Build history of the part. All positions in model axes, mm. A direction names the side the tool comes from. Coordinates: 2 decimals unless noted, no trailing zeros. Write each loop counter-clockwise with the first axis right and the second up, starting at its lowest first coordinate (ties: lowest second). Pieces come first, ordered by that corner, then holes.
Autodesk Inventor part; units mm, degrees
ref_plane "YZ Plane" through (0, 0, 0) normal (1, 0, 0) x (0, 1, 0)
ref_plane "XZ Plane" through (0, 0, 0) normal (0, 1, 0) x (-1, 0, 0)
ref_plane "XY Plane" through (0, 0, 0) normal (0, 0, 1) x (1, 0, 0)
sketch "Sketch1" plane through (0, 0, 0) normal (1, 0, 0) x (0, 1, 0)
  line L0 (0, 0) -> (25.4, 0)
  line L1 (25.4, 0) -> (25.4, -25.4)
  line L2 (25.4, -25.4) -> (0, -25.4)
  line L3 (0, -25.4) -> (0, 0)
  line L4 (23.8125, -1.5875) -> (1.5875, -1.5875)
  line L5 (1.5875, -1.5875) -> (1.5875, -23.8125)
  line L6 (1.5875, -23.8125) -> (23.8125, -23.8125)
  line L7 (23.8125, -23.8125) -> (23.8125, -1.5875)
  dimension "d0" = 25.4
  dimension "d1" = 25.4
  dimension "d2" = 1.5875
extrude "Extrusion1" add sketch "Sketch1" along normal mid plane 504.2916
chamfer "Chamfer1" distance 25.4 angle 45 1 edges at (252.1458, 0, -12.7)
chamfer "Chamfer2" distance 25.4 angle 45 1 edges at (-252.1458, 0, -12.7)
properties part number "SUP_004_TopConnectorBar" material "Aluminum 6061"
1. Saw through at C-C on x = -111. List the corners of the cut face in (y, z).
Computed values:
outline: (0, -25.4) - (25.4, -25.4) - (25.4, 0) - (0, 0) - close; hole (1.59, -23.81) - (23.81, -23.81) - (23.81, -1.59) - (1.59, -1.59) - close
2. 3-axis set-ups, long thin cutter, end or side, ignore diameter. For faces 4 (the face through (-4, 13, -1.588)), 5 (the face through (-4, 25.4, -13)): which of +Z, -Z, +X, -X, +Y, -Y reach the whole face in a straight line?
Computed values:
face 4: +X, -X
face 5: +Z, -Z, +X, -X, +Y
3. Saw through at A-A on z = -13.25. List the corners of the cut face in (x, y), plus the area to 3 significant figures.
Computed values:
outline: (-252.15, 25.4) - (-250.56, 23.81) - (250.56, 23.81) - (252.15, 25.4) - close; (-228.33, 1.59) - (-226.75, 0) - (226.75, 0) - (228.33, 1.59) - close
area: 1,520 mm2
4. Flat gauge pin, fed straight in: pin 1 (6 mm diameter, centred on y = 11.5, z = -2.5, fed in from -X). Where does the tip first touch, or does it go through?
Computed values:
pin 1: stops at x = -241.1
5. Mould opens along Y. For faces 1 (the face through (239.387, 12.641, -24.048)), 2 (the face through (-4, 23.812, -13)), 3 (the face through (-4, 13, 0)) say: +Y half, -Y half, draft (parallel to the pull), parting line (faces both ways), or undercut.
Computed values:
face 1: -Y half
face 2: undercut
face 3: draft
6. Probe line 1 along Y through (x, z) = (95.5, -17.5); line 2 along Z through (x, y) = (-15, 6.5); line 3 along X through (y, z) = (1.5, -5). List the from-to ranges inside material, lowest first.
Computed values:
line 1: y = 0 to 1.59, 23.81 to 25.4
line 2: z = -25.4 to -23.81, -1.59 to 0
line 3: x = -228.25 to 228.25
7. Saw through at B-B on y = 14. List the corners of the cut face in (x, z).
Computed values:
outline: (-240.75, -25.4) - (240.75, -25.4) - (240.75, -23.81) - (-240.75, -23.81) - close; (-240.75, -1.59) - (240.75, -1.59) - (240.75, 0) - (-240.75, 0) - close
